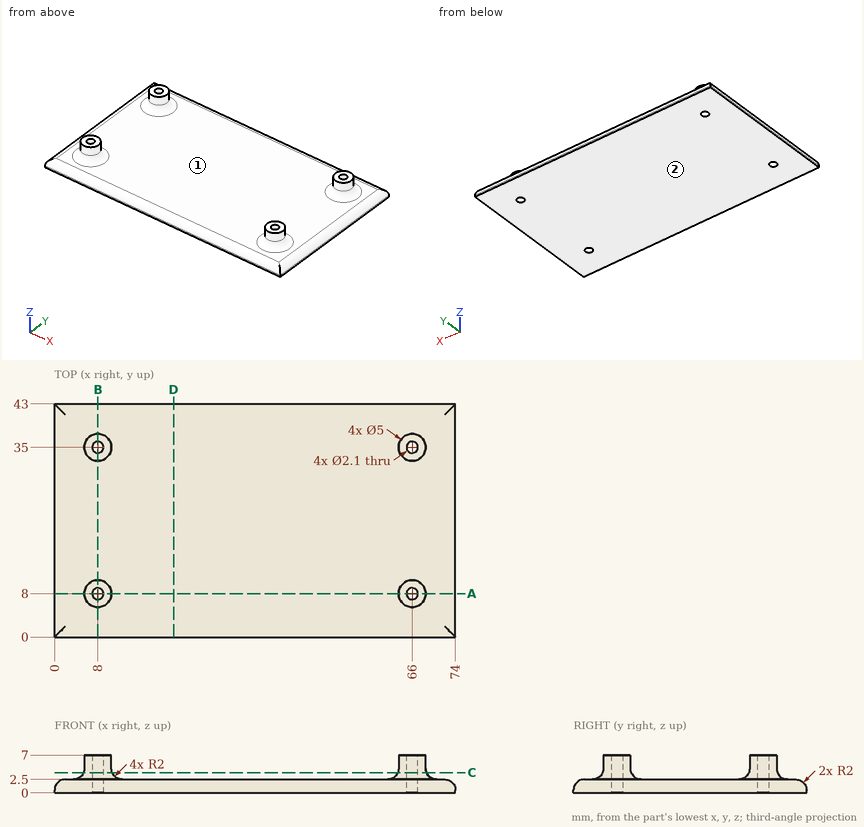
Part print with two shaded views. Sizes in mm from the minimum x, y, z corner. A direction names the side the tool comes from. Coordinates: 2 decimals unless noted, no trailing zeros. Order: outer loops, then holes, each group sorted by start corner. A loop starts at its lowest first (then second) coordinate and runs counter-clockwise, first axis right, second up. Notation, with made-up numbers: (-6, 40.5) - (42, 40.5) arc R28 ccw to (42, 60.5) - close; hole circle Ø9 at (-8.75, 57). An arc over 180 degrees is marked (long way). Answer in a Markdown table with one row per item.
1. Slice it at D-D, the plane x = 22. List the corners of the cut face in (y, z), then the cut area to 3 significant figures.
Answer:
| item | result |
|---|---|
| outline | (0, 0) - (43, 0) - (43, 0.5) arc R2 ccw to (41, 2.5) - (2, 2.5) arc R2 ccw to (0, 0.5) - close |
| area | 106 mm² |
2. Drill centre lines: L1, parallel to X at y = 35, z = 5.5; L2, parallel to Y at x = 66, z = 2; L3, parallel to Z at x = 20, y = 24. Where is each one in solid material? Low to high. Write a range as from..to.
Answer:
| item | result |
|---|---|
| L1 | 5.5..6.95, 9.05..10.5, 63.5..64.95, 67.05..68.5 |
| L2 | 0.68..6.95, 9.05..33.95, 36.05..42.32 |
| L3 | 0..2.5 |
3. 3-axis set-ups, long thin cutter, end or side, ignore diameter. For the marked faces 1 and 2: which of +Z, -Z, +X, -X, +Y, -Y reach the whole face in a straight line?
Answer:
| item | result |
|---|---|
| face 1 | +Z |
| face 2 | -Z, +X, -X, +Y, -Y |
4. Flat gauge pins, fed straight in: P1, Ø4, axis at x = 66, y = 23.5, coming from the -Z side; P2, Ø3, axis at x = 39, y = 38, coming from the +Z side. Where does each tip first touch, or does it go through?
Answer:
| item | result |
|---|---|
| P1 | z = 0 |
| P2 | z = 2.5 |
5. Slice it at B-B, the plane x = 8. List the corners of the cut face in (y, z), then the cut area to 3 significant figures.
Answer:
| item | result |
|---|---|
| outline | (0, 0) - (6.95, 0) - (6.95, 7) - (5.5, 7) - (5.5, 4.5) arc R2 cw to (3.5, 2.5) - (2, 2.5) arc R2 ccw to (0, 0.5) - close; (9.05, 0) - (33.95, 0) - (33.95, 7) - (32.5, 7) - (32.5, 4.5) arc R2 cw to (30.5, 2.5) - (12.5, 2.5) arc R2 cw to (10.5, 4.5) - (10.5, 7) - (9.05, 7) - close; (36.05, 0) - (43, 0) - (43, 0.5) arc R2 ccw to (41, 2.5) - (39.5, 2.5) arc R2 cw to (37.5, 4.5) - (37.5, 7) - (36.05, 7) - close |
| area | 125 mm² |
6. Slice it at C-C, the plane z = 3.75. List the corners of the cut face in (x, y), then the cut area to 3 significant figures.
Answer:
| item | result |
|---|---|
| outline | circle Ø5.29 at (8, 8); circle Ø5.29 at (8, 35); circle Ø5.29 at (66, 8); circle Ø5.29 at (66, 35); hole circle Ø2.1 at (8, 8); hole circle Ø2.1 at (8, 35); hole circle Ø2.1 at (66, 8); hole circle Ø2.1 at (66, 35) |
| area | 74.1 mm² |
7. Slice it at A-A, the plane y = 8. List the corners of the cut face in (x, z), then the cut area to 3 significant figures.
Answer:
| item | result |
|---|---|
| outline | (0, 0) - (6.95, 0) - (6.95, 7) - (5.5, 7) - (5.5, 4.5) arc R2 cw to (3.5, 2.5) - (2, 2.5) arc R2 ccw to (0, 0.5) - close; (9.05, 0) - (64.95, 0) - (64.95, 7) - (63.5, 7) - (63.5, 4.5) arc R2 cw to (61.5, 2.5) - (12.5, 2.5) arc R2 cw to (10.5, 4.5) - (10.5, 7) - (9.05, 7) - close; (67.05, 0) - (74, 0) - (74, 0.5) arc R2 ccw to (72, 2.5) - (70.5, 2.5) arc R2 cw to (68.5, 4.5) - (68.5, 7) - (67.05, 7) - close |
| area | 202 mm² |
